```python
from build123d import *

# Parameters (mm, degrees)
SKETCH1_W           = 330
SKETCH1_H           = 250
BOSS_EXTRUDE1_DEPTH = 6.9
SKETCH2_R           = 3
CUT_EXTRUDE1_DEPTH  = 7.9
SKETCH3_W           = 280
SKETCH3_H           = 200
CUT_EXTRUDE2_DEPTH  = 7.9
FILLET1_R           = 20
FILLET2_R           = 20


with BuildPart() as part:
    # Sketch1 → Boss-Extrude1 (new body)
    with BuildSketch(Plane(origin=(0, 0, 0), x_dir=(1, 0, 0), z_dir=(0, 1, 0))):
        Rectangle(SKETCH1_W, SKETCH1_H)
    extrude(amount=BOSS_EXTRUDE1_DEPTH)

    # Sketch2 → Cut-Extrude1 (cut, through all)
    with BuildSketch(Plane(origin=(0, 6.9, 0), x_dir=(1, 0, 0), z_dir=(0, 1, 0))):
        with Locations((-145, 105)):
            Circle(SKETCH2_R)
        with Locations((145, 105)):
            Circle(SKETCH2_R)
        with Locations((145, -105)):
            Circle(SKETCH2_R)
        with Locations((-145, -105)):
            Circle(SKETCH2_R)
    extrude(amount=-CUT_EXTRUDE1_DEPTH, mode=Mode.SUBTRACT)

    # Sketch3 → Cut-Extrude2 (cut, through all)
    with BuildSketch(Plane(origin=(0, 6.9, 0), x_dir=(1, 0, 0), z_dir=(0, 1, 0))):
        Rectangle(SKETCH3_W, SKETCH3_H)
    extrude(amount=-CUT_EXTRUDE2_DEPTH, mode=Mode.SUBTRACT)

    # Fillet1
    fillet1_edges = [part.edges().sort_by_distance(p)[0] for p in [
        (-165, 3.45, -125),
        (165, 3.45, -125),
        (165, 3.45, 125),
        (-165, 3.45, 125),
    ]]
    fillet(fillet1_edges, radius=FILLET1_R)

    # Fillet2
    fillet2_edges = [part.edges().sort_by_distance(p)[0] for p in [
        (-140, 3.45, 100),
        (-140, 3.45, -100),
        (140, 3.45, -100),
        (140, 3.45, 100),
    ]]
    fillet(fillet2_edges, radius=FILLET2_R)


solid = part.part
```
Part model, mm, in its own coordinate system. A direction names the side the tool comes from. Give positions to 0.01 mm unless a question says otherwise; leave off trailing zeros. Write each loop counter-clockwise with the first axis right and the second up, starting at its lowest first coordinate (ties: lowest second). Pieces come first, ordered by that corner, then holes. Notation, with made-up numbers: M 25.25,81 L 29.25,81 A17 ccw 29.25,100 Z; hole C -19,-28 d6. An arc over 180 degrees is marked long. Use CSV: the item, a comma, the result in double quotes.
Item 1: Which spindle directions (+Z, -Z, +X, -X, +Y, -Y) get a long thin tool onto all of the face, cutting with end or side? Do faces 1 (the face through (158.986, 3.498, -119.297)), 2 (the face through (140, 3, 1)). Say none if no direction does.
Taken from the geometry:
face 1,"-Z, +X, +Y, -Y"
face 2,"+Y, -Y"
Item 2: Slice it at C-C on y = 4.75. Write the cut outline in (x, z), plus the area to 3 significant figures.
Taken from the geometry:
outline,"M -165,-105 A20 ccw -145,-125 L 145,-125 A20 ccw 165,-105 L 165,105 A20 ccw 145,125 L -145,125 A20 ccw -165,105 Z; hole C -145,-105 d6; hole C -145,105 d6; hole M -140,-80 A20 ccw -120,-100 L 120,-100 A20 ccw 140,-80 L 140,80 A20 ccw 120,100 L -120,100 A20 ccw -140,80 Z; hole C 145,-105 d6; hole C 145,105 d6"
area,"26,400 mm²"
Item 3: Drill centre lines: probe 1 along Z at (x, y) = (-145, 5.5); probe 2 along X at (y, z) = (1.25, 105); probe 3 along X at (y, z) = (5.5, 48). Where is each one in solid material? Low to high.
Taken from the geometry:
probe 1,"z = -125 to -108, -102 to 102, 108 to 125"
probe 2,"x = -165 to -148, -142 to 142, 148 to 165"
probe 3,"x = -165 to -140, 140 to 165"
Item 4: Slice it at A-A on x = 116. Write the cut outline in (y, z).
Taken from the geometry:
outline,"M 0,-125 L 6.9,-125 L 6.9,-100 L 0,-100 Z; M 0,100 L 6.9,100 L 6.9,125 L 0,125 Z"
Item 5: Slice it at B-B on z = -75.5. Write the cut outline in (x, y).
Taken from the geometry:
outline,"M -165,0 L -140,0 L -140,6.9 L -165,6.9 Z; M 140,0 L 165,0 L 165,6.9 L 140,6.9 Z"
Item 6: Pull direction Z, two halves, no side cores. Call faces 3 (the face through (165, 3, 1)), 4 (the face through (-159.297, 3.498, -118.986)), 5 (the face through (-2, 3, 125)), 6 (the face through (-133.986, 3.402, -94.297)): +Z half, -Z half, draft (parallel to the pull), parting line (faces both ways), or undercut.
Taken from the geometry:
face 3,"draft"
face 4,"-Z half"
face 5,"+Z half"
face 6,"undercut"
